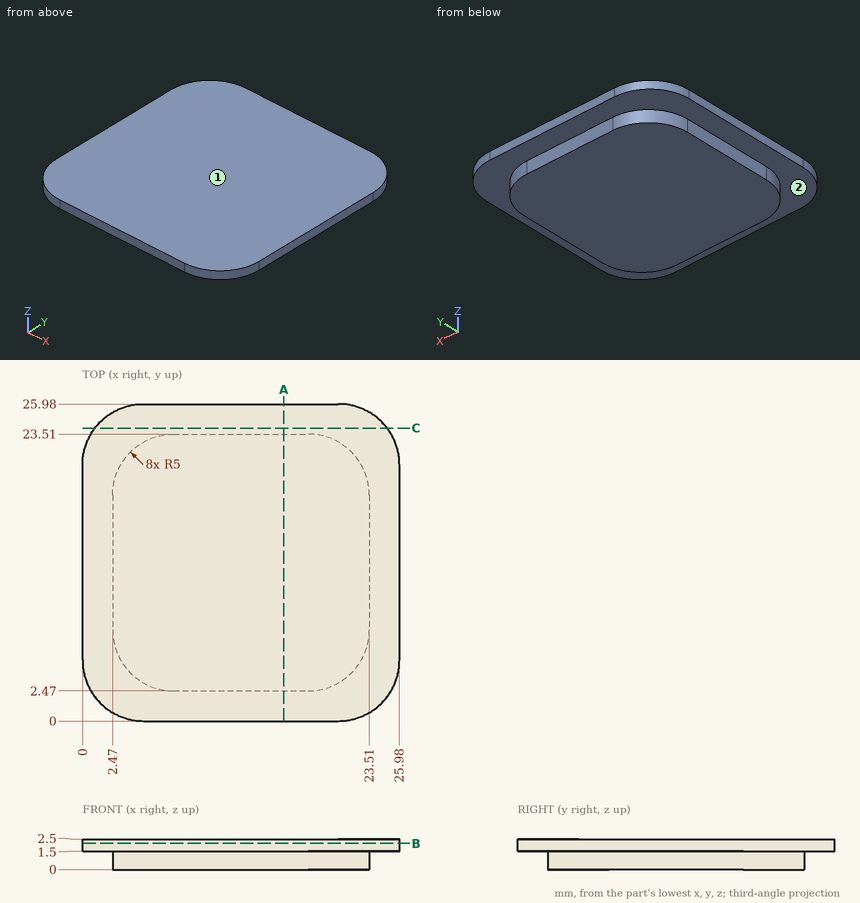
Verification items for this drawing (mm, ordinates from the low corner). A direction names the side the tool comes from. Coordinates: 2 decimals unless noted, no trailing zeros. Write each loop counter-clockwise with the first axis right and the second up, starting at its lowest first coordinate (ties: lowest second). Pieces come first, ordered by that corner, then holes. Notation, with made-up numbers: M 18,-38.5 L 26,-38.5 A11 ccw 26,-29.5 Z; hole C 72,-39 d5. An arc over 180 degrees is marked long. Answer as CSV lines item,"result".
Q1. Cross-section at A-A (x = 16.5). Record the boundary of the cut face in (y, z), then the cut area to 3 significant figures.
Check result:
outline,"M 0,1.5 L 2.47,1.5 L 2.47,0 L 23.51,0 L 23.51,1.5 L 25.98,1.5 L 25.98,2.5 L 0,2.5 Z"
area,"57.5 mm^2"
Q2. Cross-section at C-C (y = 24). Record the boundary of the cut face in (x, z), then the cut area to 3 significant figures.
Check result:
outline,"M 1.02,1.5 L 24.96,1.5 L 24.96,2.5 L 1.02,2.5 Z"
area,"23.9 mm^2"
Q3. Go/stop test with flat-tipped pins: pin 1 (1.2 mm diameter, centred on x = 14.5, z = 0.5, fed in from -Y); pin 2 (6 mm diameter, centred on x = 14, y = 12, fed in from -Z). Record where each tip stops, or that it passes through.
Check result:
pin 1,"y = 2.47"
pin 2,"z = 0"
Q4. Cross-section at B-B (z = 2.15). Record the boundary of the cut face in (x, y).
Check result:
outline,"M 0,5 A5 ccw 5,0 L 20.98,0 A5 ccw 25.98,5 L 25.98,20.98 A5 ccw 20.98,25.98 L 5,25.98 A5 ccw 0,20.98 Z"
Q5. Set-up check for the marked faces 1 and 2: record each of +Z, -Z, +X, -X, +Y, -Y from which the full face is reachable in a straight line by a thin tool's end or side.
Check result:
face 1,"+Z, +X, -X, +Y, -Y"
face 2,"-Z"
Q6. Material ranges on probe 1 along X at (y, z) = (15.5, 0.5); probe 2 along Z at (x, y) = (23.5, 4), recorded low to high. Write a range as from..to.
Check result:
probe 1,"2.47..23.51"
probe 2,"1.5..2.5"
